from build123d import *

# Parameters (mm, degrees)
BOSS_EXTRUDE1_DEPTH = 3.175


with BuildPart() as part:
    # Sketch1 → Boss-Extrude1 (new body)
    with BuildSketch(Plane.XY):
        with BuildLine():
            Line((-12.7, 0), (-25.4, 0))
            Line((-25.4, 0), (-25.4, -19.05))
            Line((-25.4, -19.05), (-19.05, -19.05))
            Line((-19.05, -19.05), (-19.05, -22.225))
            Line((-19.05, -22.225), (-6.35, -22.225))
            Line((-6.35, -22.225), (-6.35, -19.05))
            Line((-6.35, -19.05), (6.35, -19.05))
            Line((6.35, -19.05), (6.35, -22.225))
            Line((6.35, -22.225), (19.05, -22.225))
            Line((19.05, -22.225), (19.05, -19.05))
            Line((19.05, -19.05), (25.4, -19.05))
            Line((25.4, -19.05), (25.4, 0))
            Line((25.4, 0), (12.7, 0))
            ThreePointArc((12.7, 0), (0, -12.7), (-12.7, 0))
        make_face()
    extrude(amount=BOSS_EXTRUDE1_DEPTH)


solid = part.part
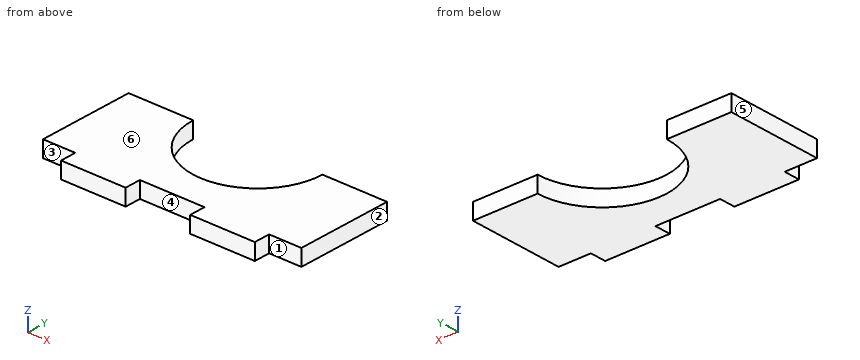
Work out the finished part from the listing and answer in its coordinate system (mm). Face numbers are marked on the shaded views. A direction names the side the tool comes from. Round coordinates to 2 decimals unless told otherwise and drop trailing zeros. Write each loop counter-clockwise with the first axis right and the second up, starting at its lowest first coordinate (ties: lowest second). Pieces come first, ordered by that corner, then holes. Notation, with made-up numbers: (-35, 30) - (2, 30) arc R26 cw to (2, 48) - close; hole circle Ø11 at (-34, 43). An arc over 180 degrees is marked (long way). Answer in a Markdown table with one row per item. Add a question column.
1. A cutting plane is placed at A-A, the plane y = -4.5. Determine the outline of the cut face in (x, z) (3 decimals), and give its area (3 significant figures).
2. Find the intervals of material crossed by line 1 along X through (y, z) = (-19.5, 2); line 2 along X through (y, z) = (-3.75, 2.1); line 3 along Y through (x, z) = (23, 2.75), in increasing order. Write a range as from..to.
3. A cutting plane is placed at C-C, the plane x = 0. Determine the outline of the cut face in (y, z) (3 decimals).
4. A cutting plane is placed at D-D, the plane y = -8.5. Determine the outline of the cut face in (x, z) (3 decimals), and give its area (3 significant figures).
5. For the marked faces 1, 2 and 3, determine the directions among +Z, -Z, +X, -X, +Y, -Y from which every point of the face is accessible in a straight line to the end or side of a thin tool.
6. A cutting plane is placed at B-B, the plane z = 2.5. Determine the outline of the cut face in (x, y) (3 decimals).
7. The mould has two halves that part along X. Classify the marked faces 4, 5 and 6: +X half, -X half, draft (parallel to the pull), parting line (faces both ways), or undercut.
8. Given pin 1 (1.5 mm diameter, centred on x = -0.5, z = 2.5, fed in from -Y); pin 2 (1.6 mm diameter, centred on y = -21, z = 1, fed in from +X); pin 3 (1.6 mm diameter, centred on y = -21, z = 1.5, fed in from -X), each flat-ended and moving along its own axis, determine where each tip first touches the part or whether it passes through.
Worked out:
| question | item | result |
|---|---|---|
| 1 | outline | (-25.4, 0) - (-11.876, 0) - (-11.876, 3.175) - (-25.4, 3.175) - close; (11.876, 0) - (25.4, 0) - (25.4, 3.175) - (11.876, 3.175) - close |
| 1 | area | 85.9 mm^2 |
| 2 | line 1 | -19.05..-6.35, 6.35..19.05 |
| 2 | line 2 | -25.4..-12.13, 12.13..25.4 |
| 2 | line 3 | -19.05..0 |
| 3 | outline | (-19.05, 0) - (-12.7, 0) - (-12.7, 3.175) - (-19.05, 3.175) - close |
| 4 | outline | (-25.4, 0) - (-9.436, 0) - (-9.436, 3.175) - (-25.4, 3.175) - close; (9.436, 0) - (25.4, 0) - (25.4, 3.175) - (9.436, 3.175) - close |
| 4 | area | 101 mm^2 |
| 5 | face 1 | +Z, -Z, +X, -Y |
| 5 | face 2 | +Z, -Z, +X, +Y, -Y |
| 5 | face 3 | +Z, -Z, -X, -Y |
| 6 | outline | (-25.4, -19.05) - (-19.05, -19.05) - (-19.05, -22.225) - (-6.35, -22.225) - (-6.35, -19.05) - (6.35, -19.05) - (6.35, -22.225) - (19.05, -22.225) - (19.05, -19.05) - (25.4, -19.05) - (25.4, 0) - (12.7, 0) arc R12.7 cw to (-12.7, 0) - (-25.4, 0) - close |
| 7 | face 4 | undercut |
| 7 | face 5 | -X half |
| 7 | face 6 | draft |
| 8 | pin 1 | y = -19.05 |
| 8 | pin 2 | x = 19.05 |
| 8 | pin 3 | x = -19.05 |
